Part model, mm, in its own coordinate system. Round coordinates to 2 decimals unless told otherwise and drop trailing zeros. Loops run counter-clockwise (first coordinate to the right, second up) from the corner with the lowest first, then second, coordinate; pieces in that order, holes last.
(1) Cut at A-A on y = 51. List the corners of the cut face in (x, z).
(2) Cut at C-C on x = -1. List the corners of the cut face in (y, z) (3 decimals).
(3) Flat gauge pins, fed straight in: pin 1 (5.5 mm diameter, centred on x = 6, z = -13, fed in from -Y); pin 2 (1.5 mm diameter, centred on y = 83.5, z = 3, fed in from +X); pin 3 (1.6 mm diameter, centred on x = 1.5, z = -31, fed in from +Y); pin 4 (6 mm diameter, centred on x = 7.5, y = 29, fed in from -Z). Where does each tip first touch, or does it go through?
(4) Cut at B-B on x = 6.5. List the corners of the cut face in (y, z) (3 decimals).
(5) Probe probe 1 along Y at (x, z) = (-1.25, 0); probe 2 along Y at (x, z) = (1.6, 0); probe 3 along Y at (x, z) = (1.25, -8). List the from-to ranges inside material, lowest first.
(6) Cut at D-D on z = 0. List the corners of the cut face in (x, y).
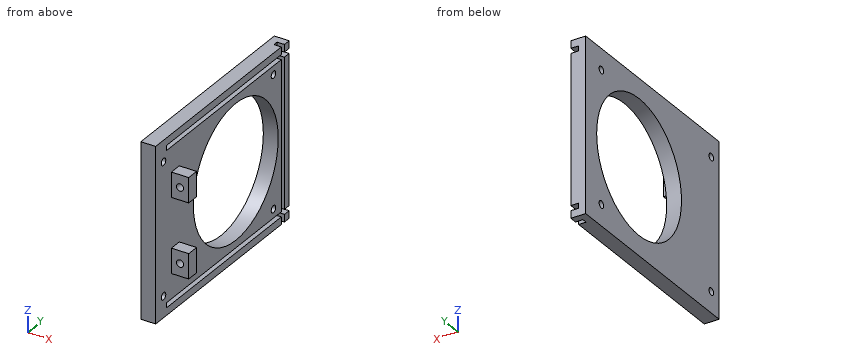
from build123d import *

# Parameters (mm, degrees)
CROQUIS1_W              = 6
CROQUIS1_H              = 70
SALIENTE_EXTRUIR1_DEPTH = 10
CROQUIS2_W              = 6
CROQUIS2_H              = 70
SALIENTE_EXTRUIR2_DEPTH = 75
CROQUIS3_W              = 2
CROQUIS3_H              = 78
CORTAR_EXTRUIR1_DEPTH   = 3
CROQUIS4_W              = 70
CROQUIS4_H              = 2
CORTAR_EXTRUIR2_DEPTH   = 3
CORTAR_EXTRUIR3_REACH   = 8
CROQUIS5_R              = 27
CROQUIS8_R              = 1.435
CORTAR_EXTRUIR5_DEPTH   = 15
MATRIZL1_COUNT          = 2
MATRIZL1_PITCH          = 70
MATRIZL1_COUNT_DIR2     = 2
MATRIZL1_PITCH_DIR2     = 53
CROQUIS12_W             = 10
CROQUIS12_H             = 5
SALIENTE_EXTRUIR3_DEPTH = 7
CROQUIS13_R             = 1.435
CORTAR_EXTRUIR10_DEPTH  = 5


with BuildPart() as part:
    # Croquis1 → Saliente-Extruir1 (new body)
    with BuildSketch(Plane(origin=(0, 0, 0), x_dir=(1, 0, 0), z_dir=(0, 1, 0))):
        Rectangle(CROQUIS1_W, CROQUIS1_H)
    extrude(amount=SALIENTE_EXTRUIR1_DEPTH)

    # Croquis2 → Saliente-Extruir2 (add)
    with BuildSketch(Plane(origin=(0, 10, 0), x_dir=(1, 0, 0), z_dir=(0, 1, 0))):
        Rectangle(CROQUIS2_W, CROQUIS2_H)
    extrude(amount=SALIENTE_EXTRUIR2_DEPTH)

    # Croquis3 → Cortar-Extruir1 (cut)
    with BuildSketch(Plane(origin=(3, 0, 0), x_dir=(0, 0, -1), z_dir=(1, 0, 0))):
        with Locations((-31, 46)):
            Rectangle(CROQUIS3_W, CROQUIS3_H)
    cortar_extruir1 = extrude(amount=-CORTAR_EXTRUIR1_DEPTH, mode=Mode.SUBTRACT)

    # Simetría1: Cortar-Extruir1 across plane
    add(cortar_extruir1.mirror(Plane.XY), mode=Mode.SUBTRACT)

    # Croquis4 → Cortar-Extruir2 (cut)
    with BuildSketch(Plane(origin=(3, 0, 0), x_dir=(0, 0, -1), z_dir=(1, 0, 0))):
        with Locations((0, 81)):
            Rectangle(CROQUIS4_W, CROQUIS4_H)
    extrude(amount=-CORTAR_EXTRUIR2_DEPTH, mode=Mode.SUBTRACT)

    # Croquis5 → Cortar-Extruir3 (cut, up to next)
    with BuildSketch(Plane(origin=(3, 0, 0), x_dir=(0, 0, -1), z_dir=(1, 0, 0)), mode=Mode.PRIVATE) as cortar_extruir3_sk1:
        with Locations((0, 51)):
            Circle(CROQUIS5_R)
    cortar_extruir3_tool1 = extrude(cortar_extruir3_sk1.sketch, amount=-CORTAR_EXTRUIR3_REACH, mode=Mode.PRIVATE) & part.part
    add(cortar_extruir3_tool1.solids().sort_by_distance((3, 51, 0))[0], mode=Mode.SUBTRACT)

    # Croquis8 → Cortar-Extruir5 (cut)
    with BuildSketch(Plane.ZY.offset(3)):
        with Locations((26.5, 75)):
            Circle(CROQUIS8_R)
    cortar_extruir5 = extrude(amount=-CORTAR_EXTRUIR5_DEPTH, mode=Mode.SUBTRACT)

    # MatrizL1: Cortar-Extruir5 2 × 2
    with Locations(*[(0, -i * MATRIZL1_PITCH, -j * MATRIZL1_PITCH_DIR2) for i in range(MATRIZL1_COUNT) for j in range(MATRIZL1_COUNT_DIR2) if (i, j) != (0, 0)]):
        add(cortar_extruir5, mode=Mode.SUBTRACT)

    # Croquis12 → Saliente-Extruir3 (add)
    with BuildSketch(Plane(origin=(3, 0, 0), x_dir=(0, 0, -1), z_dir=(1, 0, 0))):
        with Locations((-15, 12.5)):
            Rectangle(CROQUIS12_W, CROQUIS12_H)
    saliente_extruir3 = extrude(amount=SALIENTE_EXTRUIR3_DEPTH)

    # Simetría4: Saliente-Extruir3 across plane
    add(saliente_extruir3.mirror(Plane.XY))

    # Croquis13 → Cortar-Extruir10 (cut)
    with BuildSketch(Plane(origin=(0, 15, 0), x_dir=(1, 0, 0), z_dir=(0, 1, 0))):
        with Locations((6.5, -15)):
            Circle(CROQUIS13_R)
    cortar_extruir10 = extrude(amount=-CORTAR_EXTRUIR10_DEPTH, mode=Mode.SUBTRACT)

    # Simetría5: Cortar-Extruir10 across plane
    add(cortar_extruir10.mirror(Plane.XY), mode=Mode.SUBTRACT)


solid = part.part
Final values:
1. outline: (-3, -35) - (3, -35) - (3, -32) - (0, -32) - (0, -30) - (3, -30) - (3, -27) - (-3, -27) - close; (-3, 27) - (3, 27) - (3, 30) - (0, 30) - (0, 32) - (3, 32) - (3, 35) - (-3, 35) - close
2. outline: (0, -35) - (85, -35) - (85, 35) - (0, 35) - close; hole circle Ø2.87 at (5, -26.5); hole circle Ø2.87 at (5, 26.5); hole circle Ø54 at (51, 0); hole circle Ø2.87 at (75, -26.5); hole circle Ø2.87 at (75, 26.5)
3. pin 1: stops at y = 10
3. pin 2: stops at x = 3
3. pin 3: stops at y = 7
3. pin 4: passes through
4. outline: (10, -20) - (15, -20) - (15, -16.435) - (10, -16.435) - close; (10, -13.565) - (15, -13.565) - (15, -10) - (10, -10) - close; (10, 10) - (15, 10) - (15, 13.565) - (10, 13.565) - close; (10, 16.435) - (15, 16.435) - (15, 20) - (10, 20) - close
5. probe 1: y = 0 to 24, 78 to 85
5. probe 2: y = 0 to 24, 78 to 80, 82 to 85
5. probe 3: y = 0 to 25.21, 76.79 to 80, 82 to 85
6. outline: (-3, 0) - (3, 0) - (3, 24) - (-3, 24) - close; (-3, 78) - (3, 78) - (3, 80) - (0, 80) - (0, 82) - (3, 82) - (3, 85) - (-3, 85) - close
